Model file for the job. Use its own axes, mm. A direction names the side the tool comes from. Round coordinates to 2 decimals unless told otherwise and drop trailing zeros. Loops run counter-clockwise (first coordinate to the right, second up) from the corner with the lowest first, then second, coordinate; pieces in that order, holes last. Notation, with made-up numbers: M -5.5,82 L 13.5,82 A26 cw 13.5,112 Z; hole C -40,-24 d5. An arc over 180 degrees is marked long. Answer in a Markdown table with one row per item.
from build123d import *

# Parameters (mm, degrees)
F0_W     = 38.1
F0_H     = 203.2
F1_DEPTH = 3.175
F2_W     = 6.35
F2_H     = 196.85
F2_H_2   = 6.35
F2_W_2   = 25.4
F3_DEPTH = 25.4
F4_W     = 25.4
F4_H     = 152.4
F5_DEPTH = 3.176


with BuildPart() as f1:
    # F0 (on Top) → F1 (new body)
    with BuildSketch(Plane.XY):
        Rectangle(F0_W, F0_H)
    extrude(amount=F1_DEPTH)

    # F2 (on face) → F3 (join)
    with BuildSketch(Plane.XY.offset(3.175)):
        with Locations((-15.875, 3.175)):
            Rectangle(F2_W, F2_H)
        with Locations((-15.875, -98.425)):
            Rectangle(F2_W, F2_H_2)
        with Locations((0, -98.425)):
            Rectangle(F2_W_2, F2_H_2)
        with Locations((15.875, -98.425)):
            Rectangle(F2_W, F2_H_2)
        with Locations((15.875, 3.175)):
            Rectangle(F2_W, F2_H)
    extrude(amount=F3_DEPTH)

    # F4 (on face) → F5 (cut, through all)
    with BuildSketch(Plane.XY.offset(3.175)):
        Rectangle(F4_W, F4_H)
    extrude(amount=-F5_DEPTH, mode=Mode.SUBTRACT)


solid = f1.part
1. Tool access for faces 1 (the flat face through (0, -76.2, 2)), 2 (the flat face through (-14, -7, 28.575)), 3 (the flat face through (0, -95.25, 16)): list every direction of +Z, -Z, +X, -X, +Y, -Y with a clear straight run to the whole face (end or side of a thin tool).
Verdict:
| item | result |
|---|---|
| face 1 | +Z, -Z |
| face 2 | +Z, +X, -X, +Y, -Y |
| face 3 | +Z, +Y |
2. Saw through at A-A (x = -8.5). Write the cut outline in (y, z) (3 decimals).
Verdict:
| item | result |
|---|---|
| outline | M -101.6,0 L -76.2,0 L -76.2,3.175 L -95.25,3.175 L -95.25,28.575 L -101.6,28.575 Z; M 76.2,0 L 101.6,0 L 101.6,3.175 L 76.2,3.175 Z |
3. Wall check: probe 1 along X at (y, z) = (49.5, 10.5); probe 2 along Y at (x, z) = (-12, 1); probe 3 along Y at (x, z) = (-11, 8.75). Give the ranges that are in metal, low to high.
Verdict:
| item | result |
|---|---|
| probe 1 | x = -19.05 to -12.7, 12.7 to 19.05 |
| probe 2 | y = -101.6 to -76.2, 76.2 to 101.6 |
| probe 3 | y = -101.6 to -95.25 |
4. Saw through at C-C (z = 26.75). Write the cut outline in (x, y), and give its area (3 significant figures).
Verdict:
| item | result |
|---|---|
| outline | M -19.05,-101.6 L 19.05,-101.6 L 19.05,101.6 L 12.7,101.6 L 12.7,-95.25 L -12.7,-95.25 L -12.7,101.6 L -19.05,101.6 Z |
| area | 2,740 mm² |
5. Mould opens along Y. For faces 4 (the flat face through (0, -86, 3.175)), 5 (the flat face through (0, 76.2, 2)), 6 (the flat face through (0, -101.6, 14)) say: +Y half, -Y half, draft (parallel to the pull), parting line (faces both ways), or undercut.
Verdict:
| item | result |
|---|---|
| face 4 | draft |
| face 5 | undercut |
| face 6 | -Y half |
6. Saw through at B-B (y = -13). Write the cut outline in (x, z) (3 decimals), and give its area (3 significant figures).
Verdict:
| item | result |
|---|---|
| outline | M -19.05,0 L -12.7,0 L -12.7,28.575 L -19.05,28.575 Z; M 12.7,0 L 19.05,0 L 19.05,28.575 L 12.7,28.575 Z |
| area | 363 mm² |
